Verification items for the finished model (mm, model axes). A direction names the side the tool comes from. Coordinates: 2 decimals unless noted, no trailing zeros. Write each loop counter-clockwise with the first axis right and the second up, starting at its lowest first coordinate (ties: lowest second). Pieces come first, ordered by that corner, then holes. Notation, with made-up numbers: M 8,42.5 L 44,42.5 A9 ccw 44,51.5 Z; hole C -2.5,-12 d10. An arc over 180 degrees is marked long. One line per item, written item: value.
Autodesk Inventor part; units mm, degrees
ref_plane "YZ Plane" through (0, 0, 0) normal (1, 0, 0) x (0, 1, 0)
ref_plane "XZ Plane" through (0, 0, 0) normal (0, 1, 0) x (-1, 0, 0)
ref_plane "XY Plane" through (0, 0, 0) normal (0, 0, 1) x (1, 0, 0)
sketch "Sketch1" plane through (0, 0, 0) normal (1, 0, 0) x (0, 1, 0)
  line L0 (6, 6) -> (0, 6)
  line L1 (0, 6) -> (0, 0)
  line L2 (0, 0) -> (6, 0)
  line L3 (6, 0) -> (6, 6)
  line L4 (-2, 8) -> (8, 8)
  line L5 (8, 8) -> (8, -2)
  line L6 (8, -2) -> (-2, -2)
  line L7 (-2, -2) -> (-2, 8)
  dimension "d0" = 6
  dimension "d1" = 6
  dimension "d2" = 2
  dimension "d3" = 10
  dimension "d4" = 10
  dimension "d5" = 2
extrude "Extrusion1" add sketch "Sketch1" along normal blind 5
sketch "Sketch2" plane through (0, -2, -2) normal (0, -1, 0) x (1, 0, 0)
  circle A0 centre (2.5, 5) radius 2.5
  line L0 (0, 10) -> (5, 10)
  line L1 (5, 10) -> (5, 0)
  point P0 (0, 2)
  dimension "d8" = 5
  dimension "d9" = 5
  dimension "d10" = 2.5
extrude "Extrusion2" add sketch "Sketch2" along normal blind 20
fillet "Fillet1" radius 2 4 edges at (2.5, 8, 8) (2.5, 8, -2) (2.5, -2, 8) (2.5, -2, -2)
properties part number "roka2"
Item 1: Draft check along Y on faces 5 (the face through (2.54, 7.43, 7.4)), 6 (the face through (2.3, -2, 0.3)), 7 (the face through (2, 0, 3)). Enter one of: released by +Y, released by -Y, zero draft, split by the parting line, or undercut.
The answers:
face 5: released by +Y
face 6: released by -Y
face 7: undercut
Item 2: Scan lines: line 1 (Z direction, x = 2.75, y = 3.25); line 2 (Y direction, x = 0.5, z = 4); line 3 (Z direction, x = 2.6, y = -20.25). Record each from-to range of solid material in increasing order.
The answers:
line 1: z = -2 to 0, 6 to 8
line 2: y = -22 to 0, 6 to 8
line 3: z = 0.5 to 5.5
Item 3: Cross-section at B-B, the plane x = 4.5. Enter the section's corners in (y, z).
The answers:
outline: M -22,1.5 L -2,1.5 L -2,0 A2 ccw 0,-2 L 6,-2 A2 ccw 8,0 L 8,6 A2 ccw 6,8 L 0,8 A2 ccw -2,6 L -2,4.5 L -22,4.5 Z; hole M 0,0 L 6,0 L 6,6 L 0,6 Z
Item 4: Go/stop test with flat-tipped pins: P1, Ø3, axis at x = 0.5, y = -13.5, coming from the -Z side; P2, Ø3, axis at y = -5.5, z = -0.5, coming from the -X side. Record where each tip stops, or that it passes through.
The answers:
P1: stops at z = 0.55
P2: stops at x = 1
Item 5: Cross-section at D-D, the plane y = -16.75. Enter the section's corners in (x, z), and give its area (3 significant figures).
The answers:
outline: C 2.5,3 d5
area: 19.6 mm²
Item 6: Access from +Z, -Z, +X, -X, +Y, -Y to the whole of each face (thin tool, end or side, straight path). Record for faces 1 (the face through (2, 3, 0)), 2 (the face through (1, -12, 5)), 3 (the face through (2.7, -2, 5.7)), 4 (the face through (2.54, -1.43, -1.4)).
The answers:
face 1: +X, -X
face 2: -Y
face 3: +Z, -Y
face 4: -Z, +X, -X, -Y
Item 7: Cross-section at A-A, the plane y = 4.25. Enter the section's corners in (x, z).
The answers:
outline: M 0,-2 L 5,-2 L 5,0 L 0,0 Z; M 0,6 L 5,6 L 5,8 L 0,8 Z
Item 8: Cross-section at C-C, the plane z = 4.25. Enter the section's corners in (x, y).
The answers:
outline: M 0,-2 L 0.33,-2 L 0.33,-22 L 4.67,-22 L 4.67,-2 L 5,-2 L 5,0 L 0,0 Z; M 0,6 L 5,6 L 5,8 L 0,8 Z
